```python
from build123d import *

# Parameters (mm, degrees)
SKETCH_1_W           = 19
SKETCH_1_H           = 19
SKETCH_1_W_2         = 55
SKETCH_1_H_2         = 7
EXTRUDE_1_DEPTH      = 21
SKETCH_1_3_W         = 13
SKETCH_1_3_H         = 13
CUT_EXTRUDE_1_DEPTH  = 21
SKETCH_1_12_W        = 19
SKETCH_1_12_H        = 19
SKETCH_1_12_W_2      = 14.6
SKETCH_1_12_H_2      = 14.6
CUT_EXTRUDE_6_DEPTH  = 18
CUT_EXTRUDE_7_DEPTH  = 14.5
SKETCH_4_W           = 3.5
SKETCH_4_H           = 7
SKETCH_4_W_2         = 3.504900739
EXTRUDE_2_DEPTH      = 27.5
SKETCH_5_W           = 3
SKETCH_5_H           = 4
CUT_EXTRUDE_8_DEPTH  = 2.5
SKETCH_7_W           = 3
SKETCH_7_H           = 4
CUT_EXTRUDE_9_DEPTH  = 2.5
SKETCH_9_W           = 3
SKETCH_9_H           = 4
CUT_EXTRUDE_10_DEPTH = 2.5
SKETCH_10_W          = 3
SKETCH_10_H          = 4
CUT_EXTRUDE_11_DEPTH = 2.5


with BuildPart() as part:
    # Sketch 1 → Extrude 1 (new body, symmetric)
    with BuildSketch(Plane.XY):
        Rectangle(SKETCH_1_W, SKETCH_1_H)
        with Locations((0, -13)):
            Rectangle(SKETCH_1_W_2, SKETCH_1_H_2)
    extrude(amount=EXTRUDE_1_DEPTH, both=True)

    # Sketch 1_3 → Cut-Extrude 1 (cut, symmetric)
    with BuildSketch(Plane.XY):
        Rectangle(SKETCH_1_3_W, SKETCH_1_3_H)
    extrude(amount=CUT_EXTRUDE_1_DEPTH, both=True, mode=Mode.SUBTRACT)

    # Sketch 1_12 → Cut-Extrude 6 (cut, symmetric)
    with BuildSketch(Plane.XY):
        Rectangle(SKETCH_1_12_W, SKETCH_1_12_H)
        Rectangle(SKETCH_1_12_W_2, SKETCH_1_12_H_2, mode=Mode.SUBTRACT)
    extrude(amount=CUT_EXTRUDE_6_DEPTH, both=True, mode=Mode.SUBTRACT)

    # Sketch 1_13 → Cut-Extrude 7 (cut, symmetric)
    with BuildSketch(Plane.XY):
        Polygon((9.5, -9.5), (-9.5, -9.5), (-27.5, -9.5), (-27.5, -16.5), (27.5, -16.5), (27.5, -9.5), align=None)
    extrude(amount=CUT_EXTRUDE_7_DEPTH, both=True, mode=Mode.SUBTRACT)

    # Sketch 4 → Extrude 2 (add, symmetric)
    with BuildSketch(Plane(origin=(0, 0, 0), x_dir=(0, 0, -1), z_dir=(1, 0, 0))):
        with Locations((22.75, -13)):
            Rectangle(SKETCH_4_W, SKETCH_4_H)
        with Locations((-22.752450369, -13)):
            Rectangle(SKETCH_4_W_2, SKETCH_4_H)
    extrude(amount=EXTRUDE_2_DEPTH, both=True)

    # Sketch 5 → Cut-Extrude 8 (cut)
    with BuildSketch(Plane(origin=(0, 0, -24.5), x_dir=(-1, 0, 0), z_dir=(0, 0, -1))):
        Polygon((-19.28, -12.503647236), (-16.28, -12.503647236), (-16.28, -16.5), (-14.213019691, -16.5), (-14.213019691, -12.503647236), (-11.186980309, -12.503647236), (-11.186980309, -16.5), (-9.12, -16.5), (-9.12, -12.503647236), (-6.12, -12.503647236), (-6.12, -16.5), (1.038031299, -16.5), (1.038031299, -12.495586292), (4.04, -12.495586292), (4.04, -16.5), (6.12, -16.5), (6.12, -12.5), (9.12, -12.5), (9.12, -16.5), (11.198647667, -16.5), (11.198647667, -12.5), (14.201352333, -12.5), (14.201352333, -16.5), (21.36, -16.5), (21.36, -12.487022539), (24.35864906, -12.487022539), (24.35864906, -16.5), (27.5, -16.5), (27.5, -9.5), (-27.5, -9.5), (-27.5, -16.5), (-24.36, -16.5), (-24.36, -12.503647236), (-21.36, -12.503647236), (-21.36, -16.5), (-19.28, -16.5), align=None)
        with Locations((17.78, -14.493511269)):
            Rectangle(SKETCH_5_W, SKETCH_5_H, mode=Mode.SUBTRACT)
        with Locations((-2.54, -14.497793146)):
            Rectangle(SKETCH_5_W, SKETCH_5_H, mode=Mode.SUBTRACT)
    extrude(amount=-CUT_EXTRUDE_8_DEPTH, mode=Mode.SUBTRACT)

    # Sketch 7 → Cut-Extrude 9 (cut)
    with BuildSketch(Plane.XY.offset(-14.5)):
        Polygon((24.36, -16.5), (27.5, -16.5), (27.5, -9.5), (-27.5, -9.5), (-27.5, -16.5), (-24.35864906, -16.5), (-24.35864906, -12.487022539), (-21.36, -12.487022539), (-21.36, -16.5), (-14.201352333, -16.5), (-14.201352333, -12.5), (-11.198647667, -12.5), (-11.198647667, -16.5), (-9.12, -16.5), (-9.12, -12.5), (-6.12, -12.5), (-6.12, -16.5), (-4.04, -16.5), (-4.04, -12.495586292), (-1.038031299, -12.495586292), (-1.038031299, -16.5), (6.12, -16.5), (6.12, -12.503647236), (9.12, -12.503647236), (9.12, -16.5), (11.186980309, -16.5), (11.186980309, -12.503647236), (14.213019691, -12.503647236), (14.213019691, -16.5), (16.28, -16.5), (16.28, -12.503647236), (19.28, -12.503647236), (19.28, -16.5), (21.36, -16.5), (21.36, -12.503647236), (24.36, -12.503647236), align=None)
        with Locations((-17.78, -14.493511269)):
            Rectangle(SKETCH_7_W, SKETCH_7_H, mode=Mode.SUBTRACT)
        with Locations((2.54, -14.497793146)):
            Rectangle(SKETCH_7_W, SKETCH_7_H, mode=Mode.SUBTRACT)
    extrude(amount=-CUT_EXTRUDE_9_DEPTH, mode=Mode.SUBTRACT)

    # Sketch 9 → Cut-Extrude 10 (cut)
    with BuildSketch(Plane(origin=(0, 0, 14.5), x_dir=(-1, 0, 0), z_dir=(0, 0, -1))):
        Polygon((27.5, -9.5), (-27.5, -9.5), (-27.5, -16.5), (-24.36, -16.5), (-24.36, -12.503647236), (-21.36, -12.503647236), (-21.36, -16.5), (-19.28, -16.5), (-19.28, -12.503647236), (-16.28, -12.503647236), (-16.28, -16.5), (-14.213019691, -16.5), (-14.213019691, -12.503647236), (-11.186980309, -12.503647236), (-11.186980309, -16.5), (-9.12, -16.5), (-9.12, -12.503647236), (-6.12, -12.503647236), (-6.12, -16.5), (1.038031299, -16.5), (1.038031299, -12.495586292), (4.04, -12.495586292), (4.04, -16.5), (6.12, -16.5), (6.12, -12.5), (9.12, -12.5), (9.12, -16.5), (11.198647667, -16.5), (11.198647667, -12.5), (14.201352333, -12.5), (14.201352333, -16.5), (21.36, -16.5), (21.36, -12.487022539), (24.35864906, -12.487022539), (24.35864906, -16.5), (27.5, -16.5), align=None)
        with Locations((-2.54, -14.497793146)):
            Rectangle(SKETCH_9_W, SKETCH_9_H, mode=Mode.SUBTRACT)
        with Locations((17.78, -14.493511269)):
            Rectangle(SKETCH_9_W, SKETCH_9_H, mode=Mode.SUBTRACT)
    extrude(amount=-CUT_EXTRUDE_10_DEPTH, mode=Mode.SUBTRACT)

    # Sketch 10 → Cut-Extrude 11 (cut)
    with BuildSketch(Plane.XY.offset(24.504900739)):
        Polygon((27.5, -9.5), (-27.5, -9.5), (-27.5, -16.5), (-24.35864906, -16.5), (-24.35864906, -12.487022539), (-21.36, -12.487022539), (-21.36, -16.5), (-14.201352333, -16.5), (-14.201352333, -12.5), (-11.198647667, -12.5), (-11.198647667, -16.5), (-9.12, -16.5), (-9.12, -12.5), (-6.12, -12.5), (-6.12, -16.5), (-4.04, -16.5), (-4.04, -12.495586292), (-1.038031299, -12.495586292), (-1.038031299, -16.5), (6.12, -16.5), (6.12, -12.503647236), (9.12, -12.503647236), (9.12, -16.5), (11.186980309, -16.5), (11.186980309, -12.503647236), (14.213019691, -12.503647236), (14.213019691, -16.5), (16.28, -16.5), (16.28, -12.503647236), (19.28, -12.503647236), (19.28, -16.5), (21.36, -16.5), (21.36, -12.503647236), (24.36, -12.503647236), (24.36, -16.5), (27.5, -16.5), align=None)
        with Locations((-17.78, -14.493511269)):
            Rectangle(SKETCH_10_W, SKETCH_10_H, mode=Mode.SUBTRACT)
        with Locations((2.54, -14.497793146)):
            Rectangle(SKETCH_10_W, SKETCH_10_H, mode=Mode.SUBTRACT)
    extrude(amount=-CUT_EXTRUDE_11_DEPTH, mode=Mode.SUBTRACT)


solid = part.part
```
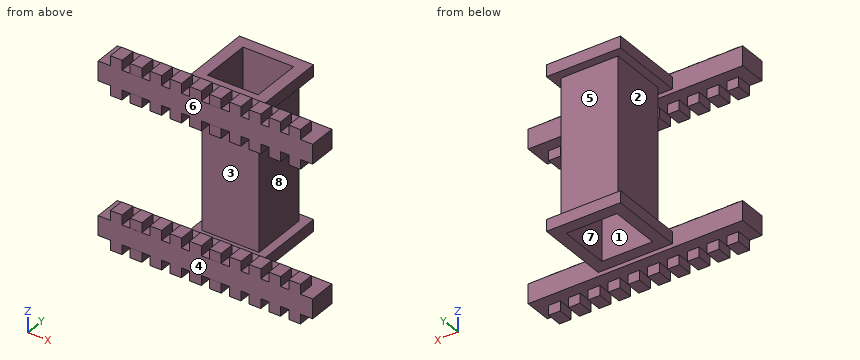
Build history of the part. All positions in model axes, mm. Face numbers are marked on the shaded views. A direction names the side the tool comes from. Round coordinates to 2 decimals unless told otherwise and drop trailing zeros. Loops run counter-clockwise (first coordinate to the right, second up) from the corner with the lowest first, then second, coordinate; pieces in that order, holes last.
Item 1: Saw through at C-C (z = -7). List the corners of the cut face in (x, y), then the cut area to 3 significant figures.
Item 2: Pin check, flat tips, straight feed: P1, Ø0.8, axis at y = -15, z = -16, coming from the -X side; P2, Ø4, axis at x = 12, z = 17.5, coming from the +Y side; P3, Ø1.2, axis at y = -14, z = -23.5, coming from the +X side; P4, Ø2, axis at x = -16, z = -13, coming from the +Y side. Stop position of each tip, or through.
Item 3: Which spindle directions (+Z, -Z, +X, -X, +Y, -Y) get a long thin tool onto all of the face, cutting with end or side? Do the marked faces 1, 2, 3, 4 and 5. Say none if no direction does.
Item 4: Drill centre lines: line 1 along X through (y, z) = (3.25, -2); line 2 along Z through (x, y) = (19.5, -11.75); line 3 along Y through (x, z) = (5.5, -20.5). Where is each one in solid material? Low to high.
Item 5: Saw through at A-A (y = -3.5). List the corners of the cut face in (x, z), then the cut area to 3 significant figures.
Item 6: Two-plate mould, pull along Y, no slides. Class the marked faces 6, 7 and 8: released by +Y, released by -Y, zero draft, split by the parting line, or undercut.
Worked answers:
1. outline: (-7.3, -7.3) - (7.3, -7.3) - (7.3, 7.3) - (-7.3, 7.3) - close; hole (-6.5, -6.5) - (6.5, -6.5) - (6.5, 6.5) - (-6.5, 6.5) - close
1. area: 44.2 mm2
2. P1: stops at x = -24.36
2. P2: stops at y = -9.5
2. P3: stops at x = 24.36
2. P4: passes through
3. face 1: +Z, -Z
3. face 2: -X, +Y
3. face 3: +X, -X
3. face 4: +Z, -Z, +X, -X, -Y
3. face 5: +X, -X, +Y
4. line 1: x = -7.3 to -6.5, 6.5 to 7.3
4. line 2: z = -22 to -17, 17 to 22
4. line 3: y = -16.5 to -6.5, 6.5 to 9.5
5. outline: (-9.5, -21) - (-6.5, -21) - (-6.5, 21) - (-9.5, 21) - (-9.5, 18) - (-7.3, 18) - (-7.3, -18) - (-9.5, -18) - close; (6.5, -21) - (9.5, -21) - (9.5, -18) - (7.3, -18) - (7.3, 18) - (9.5, 18) - (9.5, 21) - (6.5, 21) - close
5. area: 93.6 mm2
6. face 6: released by -Y
6. face 7: undercut
6. face 8: zero draft
